Check sheet for the modelled part. Datum: model origin and axes. Units: mm. Face numbers are marked on the shaded views. Round coordinates to 2 decimals unless told otherwise and drop trailing zeros. Loops run counter-clockwise (first coordinate to the right, second up) from the corner with the lowest first, then second, coordinate; pieces in that order, holes last. Notation, with made-up numbers: (0.5, 73) - (8.5, 73) arc R18 cw to (8.5, 108) - close; hole circle Ø5 at (-25.75, 21.5). An arc over 180 degrees is marked (long way). Return JSON: item names as keys, results as strings.
from build123d import *

# Parameters (mm, degrees)
F1_DEPTH = 6.35
F4_DEPTH = 25.4
F5_R     = 5.08
F6_DEPTH = 25.4


with BuildPart() as f1:
    # F0 (on Top) → F1 (new body)
    with BuildSketch(Plane.XY):
        with BuildLine():
            ThreePointArc((-21.4647859524, 13.5802416775), (-7.0694567263, -24.396368205), (25.4, 0))
            ThreePointArc((25.4, 0), (24.396368205, 7.0694567263), (21.4647859524, 13.5802416775))
            ThreePointArc((21.4647859524, 13.5802416775), (14.5838817936, 16.8865999715), (10.3111400831, 23.2129358373))
            ThreePointArc((10.3111400831, 23.2129358373), (0, 25.4), (-10.3111400831, 23.2129358373))
            ThreePointArc((-10.3111400831, 23.2129358373), (-14.5838817936, 16.8865999715), (-21.4647859524, 13.5802416775))
        make_face()
        with BuildLine():
            ThreePointArc((-9.525, 27.94), (-35.360126361, 37.277573931), (-21.4647859524, 13.5802416775))
            ThreePointArc((-21.4647859524, 13.5802416775), (-16.6019447068, 19.2233043973), (-10.3111400831, 23.2129358373))
            ThreePointArc((-10.3111400831, 23.2129358373), (-9.7228754763, 25.544005852), (-9.525, 27.94))
        make_face()
        with BuildLine():
            ThreePointArc((-10.3111400831, 23.2129358373), (-16.6019447068, 19.2233043973), (-21.4647859524, 13.5802416775))
            ThreePointArc((-21.4647859524, 13.5802416775), (-14.5838817936, 16.8865999715), (-10.3111400831, 23.2129358373))
        make_face()
        with BuildLine():
            ThreePointArc((10.3111400831, 23.2129358373), (14.5838817936, 16.8865999715), (21.4647859524, 13.5802416775))
            ThreePointArc((21.4647859524, 13.5802416775), (16.6019447068, 19.2233043973), (10.3111400831, 23.2129358373))
        make_face()
        with BuildLine():
            ThreePointArc((10.3111400831, 23.2129358373), (16.6019447068, 19.2233043973), (21.4647859524, 13.5802416775))
            ThreePointArc((21.4647859524, 13.5802416775), (33.467573931, 16.709873639), (38.735, 27.94))
            ThreePointArc((38.735, 27.94), (21.734005852, 42.3471245237), (10.3111400831, 23.2129358373))
        make_face()
    extrude(amount=F1_DEPTH)

    # F3 (on face) → F4 (cut)
    with BuildSketch(Plane.XY.offset(6.35)):
        with BuildLine():
            Line((12.2104091206, -6.8823373568), (-12.2104091206, -6.8823373568))
            ThreePointArc((-12.2104091206, -6.8823373568), (0, -18.1409484321), (12.2104091206, -6.8823373568))
        make_face()
    extrude(amount=-F4_DEPTH, mode=Mode.SUBTRACT)

    # F5 (on face) → F6 (cut)
    with BuildSketch(Plane.XY.offset(6.35)):
        with Locations((-7.62, 8.3576626432)):
            Circle(F5_R)
        with Locations((7.62, 8.3576626432)):
            Circle(F5_R)
    extrude(amount=-F6_DEPTH, mode=Mode.SUBTRACT)


solid = f1.part
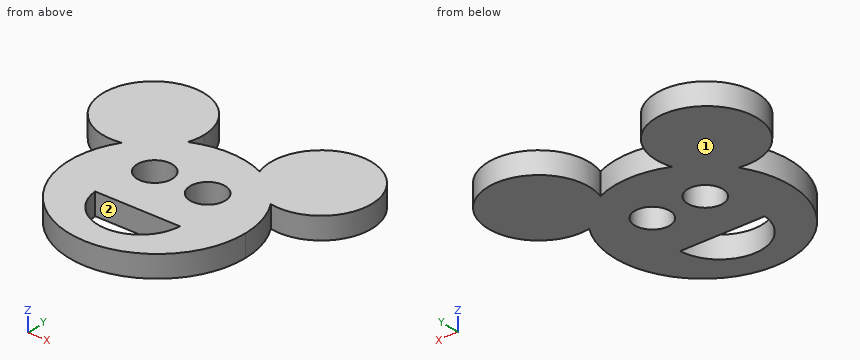
Q1. Sectioned sample at A-A (x = 0). Enter the section's corners in (y, z), plus the area to 3 significant figures.
Answer key:
{"outline": "(-25.4, 0) - (-18.14, 0) - (-18.14, 6.35) - (-25.4, 6.35) - close; (-6.88, 0) - (25.4, 0) - (25.4, 6.35) - (-6.88, 6.35) - close", "area": "251 mm²"}
Q2. Draft check along Y on the marked faces 1 and 2. Enter one of: released by +Y, released by -Y, zero draft, split by the parting line, or undercut.
Answer key:
{"face 1": "zero draft", "face 2": "undercut"}
Q3. Sectioned sample at D-D (y = 6). Enter the section's corners in (x, z).
Answer key:
{"outline": "(-24.68, 0) - (-12.12, 0) - (-12.12, 6.35) - (-24.68, 6.35) - close; (-3.12, 0) - (3.12, 0) - (3.12, 6.35) - (-3.12, 6.35) - close; (12.12, 0) - (24.68, 0) - (24.68, 6.35) - (12.12, 6.35) - close"}
Q4. Sectioned sample at C-C (z = 4). Enter the section's corners in (x, y) (3 decimals), plus the area to 3 significant figures.
Answer key:
{"outline": "(-21.465, 13.58) arc R25.4 ccw (long way) to (21.465, 13.58) arc R14.605 ccw (long way) to (10.311, 23.213) arc R25.4 ccw to (-10.311, 23.213) arc R14.605 ccw (long way) to start; hole circle Ø10.16 at (-7.62, 8.358); hole (-12.21, -6.882) arc R12.251 ccw to (12.21, -6.882) - close; hole circle Ø10.16 at (7.62, 8.358)", "area": "2,930 mm²"}
Q5. Depth check by flat-ended pin: P1, Ø1.5, axis at x = -28, z = 1, coming from the +Y side; P2, Ø8, axis at x = 7.62, y = 8.36, coming from the +Z side; P3, Ø2, axis at y = 20.5, z = 1.5, coming from the +X side; P4, Ø3, axis at y = 13, z = 3.5, coming from the +X side. Enter the tip coordinate at first touch or a pass-through.
Answer key:
{"P1": "stops at y = 42.21", "P2": "passes through", "P3": "stops at x = 37.24", "P4": "stops at x = 29.85"}
Q6. Scan lines: probe 1 along Y at (x, z) = (-0.5, 4.25); probe 2 along X at (y, z) = (27.5, 3.25); probe 3 along Y at (x, z) = (-7.62, 2.5). Record each from-to range of solid material in increasing order. Write a range as [from, to].
Answer key:
{"probe 1": "y = [-25.4, -18.13], [-6.88, 25.4]", "probe 2": "x = [-38.73, -9.53], [9.53, 38.73]", "probe 3": "y = [-24.23, -15.48], [-6.88, 3.28], [13.44, 24.23]"}
Q7. Sectioned sample at B-B (y = 35). Enter the section's corners in (x, z).
Answer key:
{"outline": "(-36.92, 0) - (-11.34, 0) - (-11.34, 6.35) - (-36.92, 6.35) - close; (11.34, 0) - (36.92, 0) - (36.92, 6.35) - (11.34, 6.35) - close"}
